```python
from build123d import *

# Parameters (mm, degrees)
SKETCH1_W               = 5
SKETCH1_H               = 5
SKETCH1_R               = 0.95
CENTER_DEPTH            = 1.3
RIGHTSIDE_START         = 1.3
SKETCH1_2_W             = 5
SKETCH1_2_H             = 5
SKETCH1_2_R             = 0.95
RIGHTSIDE_DEPTH         = 1.2
LEFTSIDE_START          = -1.3
SKETCH1_3_W             = 5
SKETCH1_3_H             = 5
SKETCH1_3_R             = 0.95
LEFTSIDE_DEPTH          = 1.2
SKETCH3_W               = 5
SKETCH3_H               = 5
BOSS_EXTRUDE4_DEPTH     = 47.5
CUT_EXTRUDE1_DEPTH      = 5
CIRPATTERN2_COUNT       = 6
CIRPATTERN3_COUNT       = 3
CIRPATTERN4_START       = -44.601270189
CIRPATTERN4_OUTLINE_W   = 5
CIRPATTERN4_OUTLINE_H   = 5
CIRPATTERN4_OUTLINE_R   = 0.95
CIRPATTERN4_DEPTH       = 2.6
CIRPATTERN4_2_OUTLINE_W = 5
CIRPATTERN4_2_OUTLINE_H = 5
CIRPATTERN4_2_OUTLINE_R = 0.95
CIRPATTERN4_2_DEPTH     = 2.6
CIRPATTERN4_START_2     = -1.3
CIRPATTERN4_3_OUTLINE_W = 5
CIRPATTERN4_3_OUTLINE_H = 5
CIRPATTERN4_3_OUTLINE_R = 0.95
CIRPATTERN4_3_DEPTH     = 2.6
SKETCH5_W               = 5
SKETCH5_H               = 2.6
CUT_EXTRUDE2_DEPTH      = 5


# Read off the part's stored shape, not the designer's step: CirPattern4
with BuildPart() as part:
    # Sketch1 → Center (new, symmetric)
    with BuildSketch(Plane(origin=(0, 0, 0), x_dir=(1, 0, 0), z_dir=(0, 1, 0))):
        Rectangle(SKETCH1_W, SKETCH1_H)
        with Locations(Location((0, 0, 0), (0, 0, 270))):
            Circle(SKETCH1_R, mode=Mode.SUBTRACT)
    extrude(amount=CENTER_DEPTH, both=True)

    # Sketch5 → Cut-Extrude2 (cut)
    with BuildSketch(Plane(origin=(2.5, 0, 0), x_dir=(0, 0, -1), z_dir=(1, 0, 0))):
        Rectangle(SKETCH5_W, SKETCH5_H)
    extrude(amount=-CUT_EXTRUDE2_DEPTH, mode=Mode.SUBTRACT)


with BuildPart() as body_2:
    # Sketch1<2> → RightSide (new body)
    with BuildSketch(Plane(origin=(0, 0, 0), x_dir=(1, 0, 0), z_dir=(0, 1, 0)).offset(RIGHTSIDE_START)):
        Rectangle(SKETCH1_2_W, SKETCH1_2_H)
        with Locations(Location((0, 0, 0), (0, 0, 270))):
            Circle(SKETCH1_2_R, mode=Mode.SUBTRACT)
    extrude(amount=RIGHTSIDE_DEPTH)


with BuildPart() as body_3:
    # Sketch1<3> → LeftSide (new body)
    with BuildSketch(Plane(origin=(0, 0, 0), x_dir=(1, 0, 0), z_dir=(0, 1, 0)).offset(LEFTSIDE_START)):
        Rectangle(SKETCH1_3_W, SKETCH1_3_H)
        with Locations(Location((0, 0, 0), (0, 0, 270))):
            Circle(SKETCH1_3_R, mode=Mode.SUBTRACT)
    extrude(amount=-LEFTSIDE_DEPTH)


with BuildPart() as body_4:
    # Sketch3 → Boss-Extrude4 (new body)
    with BuildSketch(Plane.ZY.offset(2.5)):
        Rectangle(SKETCH3_W, SKETCH3_H)
    extrude(amount=BOSS_EXTRUDE4_DEPTH)

    # Sketch4 → Cut-Extrude1 (cut)
    with BuildSketch(Plane.XY.offset(-2.5)):
        Polygon((-50, 0), (-50, -2.5), (-45.669872981, -2.5), align=None)
        Polygon((-50, 2.5), (-50, 0), (-45.669872981, 2.5), align=None)
    extrude(amount=CUT_EXTRUDE1_DEPTH, mode=Mode.SUBTRACT)


with BuildPart() as cirpattern2_1:
    # CirPattern2: pattern copy
    add(body_4.part.rotate(Axis((-50, 0, 0), (0, 0, 1)), 1 * 360 / CIRPATTERN2_COUNT))


with BuildPart() as cirpattern2_2:
    # CirPattern2: pattern copy
    add(body_4.part.rotate(Axis((-50, 0, 0), (0, 0, 1)), 2 * 360 / CIRPATTERN2_COUNT))


with BuildPart() as cirpattern2_3:
    # CirPattern2: pattern copy
    add(body_4.part.rotate(Axis((-50, 0, 0), (0, 0, 1)), 3 * 360 / CIRPATTERN2_COUNT))


with BuildPart() as cirpattern2_4:
    # CirPattern2: pattern copy
    add(body_4.part.rotate(Axis((-50, 0, 0), (0, 0, 1)), 4 * 360 / CIRPATTERN2_COUNT))


with BuildPart() as cirpattern2_5:
    # CirPattern2: pattern copy
    add(body_4.part.rotate(Axis((-50, 0, 0), (0, 0, 1)), 5 * 360 / CIRPATTERN2_COUNT))


with BuildPart() as cirpattern3_1:
    # CirPattern3: pattern copy
    add(body_3.part.rotate(Axis((-50, 0, 0), (0, 0, 1)), 1 * 360 / CIRPATTERN3_COUNT))


with BuildPart() as cirpattern3_2:
    # CirPattern3: pattern copy
    add(body_3.part.rotate(Axis((-50, 0, 0), (0, 0, 1)), 2 * 360 / CIRPATTERN3_COUNT))


with BuildPart() as cirpattern3_3:
    # CirPattern3: pattern copy
    add(body_2.part.rotate(Axis((-50, 0, 0), (0, 0, 1)), 1 * 360 / CIRPATTERN3_COUNT))


with BuildPart() as cirpattern3_4:
    # CirPattern3: pattern copy
    add(body_2.part.rotate(Axis((-50, 0, 0), (0, 0, 1)), 2 * 360 / CIRPATTERN3_COUNT))


with BuildPart() as body_14:
    # CirPattern4 outline → CirPattern4 (new body)
    with BuildSketch(Plane(origin=(0, 0, 0), x_dir=(0.49999999999999767, 0.86602540378444, 0), z_dir=(0.8660254037844399, -0.49999999999999795, 0)).offset(CIRPATTERN4_START)):
        with Locations((25, 0)):
            Rectangle(CIRPATTERN4_OUTLINE_W, CIRPATTERN4_OUTLINE_H)
        with Locations((25, 0)):
            Circle(CIRPATTERN4_OUTLINE_R, mode=Mode.SUBTRACT)
    extrude(amount=CIRPATTERN4_DEPTH)


with BuildPart() as body_15:
    # CirPattern4 2 outline → CirPattern4 2 (new body)
    with BuildSketch(Plane(origin=(0, 0, 0), x_dir=(0.5000000000000098, -0.8660254037844329, 0), z_dir=(0.8660254037844329, 0.50000000000001, 0)).offset(CIRPATTERN4_START)):
        with Locations((25, 0)):
            Rectangle(CIRPATTERN4_2_OUTLINE_W, CIRPATTERN4_2_OUTLINE_H)
        with Locations((25, 0)):
            Circle(CIRPATTERN4_2_OUTLINE_R, mode=Mode.SUBTRACT)
    extrude(amount=CIRPATTERN4_2_DEPTH)


with BuildPart() as body_16:
    # CirPattern4 3 outline → CirPattern4 3 (new body)
    with BuildSketch(Plane(origin=(0, 0, 0), x_dir=(1, 0, 0), z_dir=(0, 1, 0)).offset(CIRPATTERN4_START_2)):
        with Locations((-100, 0)):
            Rectangle(CIRPATTERN4_3_OUTLINE_W, CIRPATTERN4_3_OUTLINE_H)
        with Locations((-100, 0)):
            Circle(CIRPATTERN4_3_OUTLINE_R, mode=Mode.SUBTRACT)
    extrude(amount=CIRPATTERN4_3_DEPTH)


with BuildPart() as cirpattern2_5_1:
    add(cirpattern2_5.part)

    # Combine1: union CirPattern2_3, CirPattern2_4, body 16, CirPattern3_2, CirPattern3_4, body 15
    add(cirpattern2_3.part)
    add(cirpattern2_4.part)
    add(body_16.part)
    add(cirpattern3_2.part)
    add(cirpattern3_4.part)
    add(body_15.part)

    # Combine3: cut CirPattern3_3, body 14, CirPattern2_1, body 4, body 2, CirPattern2_2, body 3, CirPattern3_1
    add(cirpattern3_3.part, mode=Mode.SUBTRACT)
    add(body_14.part, mode=Mode.SUBTRACT)
    add(cirpattern2_1.part, mode=Mode.SUBTRACT)
    add(body_4.part, mode=Mode.SUBTRACT)
    add(body_2.part, mode=Mode.SUBTRACT)
    add(cirpattern2_2.part, mode=Mode.SUBTRACT)
    add(body_3.part, mode=Mode.SUBTRACT)
    add(cirpattern3_1.part, mode=Mode.SUBTRACT)


solid = cirpattern2_5_1.part
```
Geometry: final body of the model. Coordinates: model frame, mm. A direction names the side the tool comes from. Round coordinates to 2 decimals unless told otherwise and drop trailing zeros. Order: outer loops, then holes, each group sorted by start corner. A loop starts at its lowest first (then second) coordinate and runs counter-clockwise, first axis right, second up. Notation, with made-up numbers: (32.5, 84) - (37.5, 84) arc R17 ccw to (37.5, 114) - close; hole circle Ø5 at (30.25, 33). An arc over 180 degrees is marked (long way). Write item = value, one per line. Start each with the question number.
Q1. Access query for faces 5 (the flat face through (-76, -2.5, 0)), 6 (the flat face through (-101.15, 1.3, -0.04)), 7 (the flat face through (-61.874, -25.566, -0.035)). Directions: +Z, -Z, +X, -X, +Y, -Y. A direction counts if a zero-diameter tool reaches every point of the face in a straight line with its end or side. Return the directions, or none.
Q2. Cut plane D-D on x = -35. Return the cut outline in (y, z).
Q3. Pin query (flat end, axial travel): pin 1 (3 mm diameter, centred on y = -8.5, z = 2, fed in from +X); pin 2 (2.5 mm diameter, centred on x = -69, z = 0.5, fed in from -Y); pin 3 (1 mm diameter, centred on y = 2, z = -0.5, fed in from -X). Return the tip coordinate at first contact, or that it passes through.
Q4. Cut plane A-A on x = -100. Return the cut outline in (y, z).
Q5. Cut plane C-C on z = 0. Give the number of separate pieces and of enclosed holes in the cut face, and give its area (3 significant figures).
Q6. Cut plane B-B on y = -27. Return the cut outline in (x, z), and give its area (3 significant figures).
Q7. Pull-direction query (Z, two-part tool) for faces 1 (the flat face through (-73.857, -43.921, -1.146)), 2 (the cylindrical face through (-76.174, -41.552, -0.206)), 3 (the cylindrical face through (-73.683, -44.803, -0.7)), 4 (the flat face through (-58, -14, -2.5)); classes: +Z half, -Z half, draft (parallel to the pull), parting line (faces both ways), or undercut.
Q8. Ray query, line 1 (Z direction, x = -100, y = -0.5); line 2 (X direction, y = 0, z = 0); line 3 (Y direction, x = -75, z = 0.5). Return the intervals inside material, ascending. Write a range as from..to.
Outcome:
q1.face_5 = +Z, -Z, -X
q1.face_6 = +Z, -Z, -X, +Y
q1.face_7 = +Z, -Z, -Y
q2.outline = (-30.98, -2.5) - (-20.98, -2.5) - (-20.98, 2.5) - (-30.98, 2.5) - close
q3.pin_1 = -41.34
q3.pin_2 = -40.07
q3.pin_3 = -97.5
q4.outline = (-1.3, -2.5) - (1.3, -2.5) - (1.3, -0.95) - (-1.3, -0.95) - close; (-1.3, 0.95) - (1.3, 0.95) - (1.3, 2.5) - (-1.3, 2.5) - close
q5.separate_pieces = 5
q5.enclosed_holes = 0
q5.area = 704 mm^2
q6.outline = (-68.48, -2.5) - (-62.7, -2.5) - (-62.7, 2.5) - (-68.48, 2.5) - close; (-37.3, -2.5) - (-31.52, -2.5) - (-31.52, 2.5) - (-37.3, 2.5) - close
q6.area = 57.7 mm^2
q7.face_1 = draft
q7.face_2 = undercut
q7.face_3 = undercut
q7.face_4 = -Z half
q8.line_1 = -2.5..-0.95, 0.95..2.5
q8.line_2 = -102.5..-100.95, -99.05..-50
q8.line_3 = -46.19..-45.9, -40.7..-38.3, -2.5..2.5
